Build history of the part. All positions in model axes, mm. Coordinates: 2 decimals unless noted, no trailing zeros. Order: outer loops, then holes, each group sorted by start corner. A loop starts at its lowest first (then second) coordinate and runs counter-clockwise, first axis right, second up. Notation, with made-up numbers: M 5.25,87 L 45.25,87 A16 ccw 45.25,95 Z; hole C -25,-40 d11. An arc over 180 degrees is marked long. Write item = value, one per line. Start each with the question number.
Q1. Band-saw the part on A-A on z = 58. Write the cut outline in (x, y) (3 decimals), plus the area to 3 significant figures.
Q2. Drill centre lines: probe 1 along X at (y, z) = (-26.75, 257); probe 2 along Y at (x, z) = (82, 64.5) (3 decimals); probe 3 along Z at (x, y) = (92, -25.75). Where is each one in solid material? Low to high.
Q3. Pull direction X, two halves, no side cores. Call faces 1 (the face through (111.76, -14, 175)), 2 (the face through (70, -24.765, 168)), 3 (the face through (25, -27.94, 162)): released by +X, released by -X, zero draft, split by the parting line, or undercut.
Q4. Pin check, flat tip, straight feed: P1, Ø11.5, axis at x = 75, z = 192.5, coming from the -Y side (3 decimals). Stop position of the tip, or through.
Q5. Band-saw the part on C-C on y = -15.25. Write the cut outline in (x, z).
```python
from build123d import *

# Parameters (mm, degrees)
F0_W     = 111.76
F0_H     = 27.94
F1_DEPTH = 355.6
F2_SIZE  = 27.93999
F3_W     = 38.1
F3_H     = 27.93999
F3_H_2   = 327.66001
F4_DEPTH = 3.175


# Not quite as in the source:
# - a fillet or chamfer is up to 0.001 mm smaller than in the source, because OpenCascade refuses the exact size


with BuildPart() as f1:
    # F0 (on Top) → F1 (new body)
    with BuildSketch(Plane.XY):
        with Locations((55.88, -13.97)):
            Rectangle(F0_W, F0_H)
    extrude(amount=F1_DEPTH)

    # F2 (size 27.94 in the source; OpenCascade refuses exactly that, so slightly less here)
    f2_edges = [f1.edges().sort_by_distance(p)[0] for p in [
        (55.88, -27.94, 355.6),
    ]]
    chamfer(f2_edges, length=F2_SIZE)

    # F3 (on face) → F4 (cut)
    with BuildSketch(Plane.XZ.offset(27.94)):
        with Locations((69.85, 341.630005)):
            Rectangle(F3_W, F3_H)
        with Locations((69.85, 163.830005)):
            Rectangle(F3_W, F3_H_2)
    extrude(amount=-F4_DEPTH, mode=Mode.SUBTRACT)


solid = f1.part
```
Recorded:
q1.outline = M 0,-27.94 L 50.8,-27.94 L 50.8,-24.765 L 88.9,-24.765 L 88.9,-27.94 L 111.76,-27.94 L 111.76,0 L 0,0 Z
q1.area = 3,000 mm2
q2.probe_1 = 0 to 50.8, 88.9 to 111.76
q2.probe_2 = -24.765 to 0
q2.probe_3 = 0 to 329.85
q3.face_1 = released by +X
q3.face_2 = undercut
q3.face_3 = zero draft
q4.P1 = -24.765
q5.outline = M 0,0 L 111.76,0 L 111.76,340.35 L 0,340.35 Z
